Design review of the part built by this model. Coordinates are the model's own, in mm. A direction names the side the tool comes from. Give positions to 0.01 mm unless a question says otherwise; leave off trailing zeros. Write each loop counter-clockwise with the first axis right and the second up, starting at its lowest first coordinate (ties: lowest second). Pieces come first, ordered by that corner, then holes. Notation, with made-up numbers: (-21, 24) - (37, 24) arc R26 ccw to (37, 40) - close; hole circle Ø1 at (0.25, -12.75). An arc over 180 degrees is marked (long way). Write each question's results on one line, items separated by ' | '. Start each with the question number.
from build123d import *

# Parameters (mm, degrees)
BOSS_EXTRUDE1_DEPTH     = 20
CUT_EXTRUDE1_DEPTH      = 57
CUT_EXTRUDE2_START      = -57
CUT_EXTRUDE2_DEPTH      = 57
SKETCH12_W              = 70.48528137
SKETCH12_H              = 6
CUT_EXTRUDE3_DEPTH      = 20
CUT_EXTRUDE4_DEPTH      = 104.740847077
CUT_EXTRUDE4_DEPTH_BACK = 15
SKETCH12_7_OUTSIDE_W    = 149.586
SKETCH12_7_OUTSIDE_H    = 49.586
SKETCH12_7_OUTSIDE_W_2  = 70.48528137
SKETCH12_7_OUTSIDE_H_2  = 3
SKETCH16_W              = 25.2
SKETCH16_H              = 5
CUT_EXTRUDE8_DEPTH      = 57
SKETCH18_R              = 1.4
CUT_EXTRUDE11_DEPTH     = 10
FILLET2_R               = 1
FILLET3_R               = 1.5
SKETCH20_W              = 25.2
SKETCH20_H              = 5
CUT_EXTRUDE12_DEPTH     = 57
FILLET5_R               = 3
FILLET6_R               = 4
SKETCH21_R              = 1.4
CUT_EXTRUDE13_DEPTH     = 20


with BuildPart() as part:
    # Sketch2 → Boss-Extrude1 (new body)
    with BuildSketch(Plane(origin=(0, 0, 0), x_dir=(1, 0, 0), z_dir=(0, 1, 0))):
        Polygon((-41.659950522, -21.859673837), (-41.659950522, -66.859673837), (78.340049478, -66.859673837), (78.340049478, -21.859673837), (53.582690163, -21.859673837), (53.582690163, -1.859673837), (-16.902591207, -1.859673837), (-16.902591207, -21.859673837), align=None)
    extrude(amount=BOSS_EXTRUDE1_DEPTH)

    # Sketch3 → Cut-Extrude1 (cut)
    with BuildSketch(Plane(origin=(78.340049478, 0, 0), x_dir=(0, 0, -1), z_dir=(1, 0, 0))):
        with BuildLine():
            ThreePointArc((-55.925139673, 20), (-46.912626096, 2.661343883), (-31.759673837, 15))
            ThreePointArc((-31.759673837, 15), (-32.02101772, 17.552952259), (-32.794208001, 20))
            Line((-32.794208001, 20), (-55.925139673, 20))
        make_face()
        with BuildLine():
            Line((-55.925139673, 20), (-32.794208001, 20))
            ThreePointArc((-32.794208001, 20), (-44.359673837, 27.6), (-55.925139673, 20))
        make_face()
    extrude(amount=-CUT_EXTRUDE1_DEPTH, mode=Mode.SUBTRACT)

    # Sketch5 → Cut-Extrude2 (cut)
    with BuildSketch(Plane.ZY.offset(41.659950522).offset(CUT_EXTRUDE2_START)):
        with BuildLine():
            ThreePointArc((32.794208001, 20), (41.806721579, 2.661343883), (56.959673837, 15))
            ThreePointArc((56.959673837, 15), (56.698329954, 17.552952259), (55.925139673, 20))
            Line((55.925139673, 20), (32.794208001, 20))
        make_face()
        with BuildLine():
            Line((32.794208001, 20), (55.925139673, 20))
            ThreePointArc((55.925139673, 20), (44.359673837, 27.6), (32.794208001, 20))
        make_face()
    extrude(amount=CUT_EXTRUDE2_DEPTH, mode=Mode.SUBTRACT)

    # Sketch12 → Cut-Extrude3 (cut)
    with BuildSketch(Plane(origin=(0, 0, 1.859673837), x_dir=(-1, 0, 0), z_dir=(0, 0, -1))):
        with Locations((-18.340049478, 17)):
            Rectangle(SKETCH12_W, SKETCH12_H)
    extrude(amount=-CUT_EXTRUDE3_DEPTH, mode=Mode.SUBTRACT)

    # Sketch12_7 outside → Cut-Extrude4 (cut, two sides: drawn at the far end of the back side and taken through both)
    with BuildSketch(Plane(origin=(0, 0, 1.859673837), x_dir=(-1, 0, 0), z_dir=(0, 0, -1)).offset(-CUT_EXTRUDE4_DEPTH_BACK)):
        with Locations((-18.34, 10)):
            Rectangle(SKETCH12_7_OUTSIDE_W, SKETCH12_7_OUTSIDE_H)
        with Locations((-18.340049478, 1.5)):
            Rectangle(SKETCH12_7_OUTSIDE_W_2, SKETCH12_7_OUTSIDE_H_2, mode=Mode.SUBTRACT)
        with Locations((-18.340049478, 12.5)):
            Rectangle(SKETCH12_7_OUTSIDE_W_2, SKETCH12_7_OUTSIDE_H_2, mode=Mode.SUBTRACT)
    extrude(amount=CUT_EXTRUDE4_DEPTH + CUT_EXTRUDE4_DEPTH_BACK, mode=Mode.SUBTRACT)

    # Sketch16 → Cut-Extrude8 (cut)
    with BuildSketch(Plane.ZY.offset(41.659950522)):
        with Locations((44.359673837, 17.5)):
            Rectangle(SKETCH16_W, SKETCH16_H)
    extrude(amount=-CUT_EXTRUDE8_DEPTH, mode=Mode.SUBTRACT)

    # Sketch18 → Cut-Extrude11 (cut)
    with BuildSketch(Plane(origin=(0, 20, 0), x_dir=(1, 0, 0), z_dir=(0, 1, 0))):
        with Locations(Location((-31.659950522, -26.259673837, 0), (0, 0, 270))):
            Circle(SKETCH18_R)
        with Locations(Location((-1.659950522, -26.259673837, 0), (0, 0, 90))):
            Circle(SKETCH18_R)
        with Locations(Location((-1.659950522, -62.459673837, 0), (0, 0, 270))):
            Circle(SKETCH18_R)
        with Locations(Location((-31.659950522, -62.459673837, 0), (0, 0, 90))):
            Circle(SKETCH18_R)
        with Locations(Location((38.340049478, -62.459673837, 0), (0, 0, 90))):
            Circle(SKETCH18_R)
        with Locations(Location((68.340049478, -62.459673837, 0), (0, 0, 270))):
            Circle(SKETCH18_R)
        with Locations(Location((38.340049478, -26.259673837, 0), (0, 0, 270))):
            Circle(SKETCH18_R)
        with Locations(Location((68.340049478, -26.259673837, 0), (0, 0, 90))):
            Circle(SKETCH18_R)
    extrude(amount=-CUT_EXTRUDE11_DEPTH, mode=Mode.SUBTRACT)

    # Fillet2
    fillet2_edges = [part.edges().sort_by_distance(p)[0] for p in [
        (18.340049478, 11, 16.859673837),
        (18.340049478, 3, 16.859673837),
    ]]
    fillet(fillet2_edges, radius=FILLET2_R)

    # Fillet3
    fillet3_edges = [part.edges().sort_by_distance(p)[0] for p in [
        (18.340049478, 11, 1.859673837),
        (18.340049478, 3, 1.859673837),
    ]]
    fillet(fillet3_edges, radius=FILLET3_R)

    # Sketch20 → Cut-Extrude12 (cut)
    with BuildSketch(Plane(origin=(78.340049478, 0, 0), x_dir=(0, 0, -1), z_dir=(1, 0, 0))):
        with Locations((-44.359673837, 17.5)):
            Rectangle(SKETCH20_W, SKETCH20_H)
    extrude(amount=-CUT_EXTRUDE12_DEPTH, mode=Mode.SUBTRACT)

    # Fillet5
    fillet5_edges = [part.edges().sort_by_distance(p)[0] for p in [
        (-41.659950522, 10, 21.859673837),
        (-41.659950522, 10, 66.859673837),
        (78.340049478, 10, 66.859673837),
        (78.340049478, 10, 21.859673837),
    ]]
    fillet(fillet5_edges, radius=FILLET5_R)

    # Fillet6
    fillet6_edges = [part.edges().sort_by_distance(p)[0] for p in [
        (-16.902591207, 7, 21.859673837),
        (53.582690163, 7, 21.859673837),
        (18.340049478, 14, 21.859673837),
    ]]
    fillet(fillet6_edges, radius=FILLET6_R)

    # Sketch21 → Cut-Extrude13 (cut)
    with BuildSketch(Plane(origin=(0, 14, 0), x_dir=(1, 0, 0), z_dir=(0, 1, 0))):
        with Locations(Location((38.340049478, -9.359673837, 0), (0, 0, 270))):
            Circle(SKETCH21_R)
        with Locations(Location((-1.659950522, -9.359673837, 0), (0, 0, 270))):
            Circle(SKETCH21_R)
    extrude(amount=-CUT_EXTRUDE13_DEPTH, mode=Mode.SUBTRACT)


solid = part.part
Q1. Add section C-C on z = 50. State the section outline as (x, y) points, plus the area to 3 significant figures.
Q2. For line 1 along Z through (x, y) = (68.5, 15); line 2 along Z through (x, y) = (38, 16.75); line 3 along Z through (x, y) = (30.5, 8), list the stretches that pass through material, from the lowest coordinate up. Write a range as [from, to].
Q3. Add section A-A on z = 6. State the section outline as (x, y) points, plus the area to 3 significant figures.
Q4. Insertion check: P1, Ø1.7, axis at x = 38.34, z = 9.36, coming from the -Y side (3 decimals); P2, Ø6, axis at y = 11.5, z = 39, coming from the +X side; P3, Ø10, axis at x = 38, y = 7, coming from the -Z side; P4, Ø2, axis at y = 15.5, z = 35.5, coming from the -X side. Each pin has a flat end and moves straight along its axis. Give the tip position at first contact, or say it passes through.
Q5. Add section B-B on x = 22.5. State the section outline as (y, z) points, plus the area to 3 significant figures.
Q6. The part is to be moulded in two halves that separate along Z. For faces 1 (the face through (50, 17, 31.76)), 2 (the face through (-18.105, 7.126, 20.719)), 3 (the face through (77.48, 10.14, 65.96)), say which applies: +Z half, -Z half, draft (parallel to the pull), parting line (faces both ways), or undercut.
Q7. Machinability: for faces 4 (the face through (53.583, 12, 10)), 5 (the face through (39.7, 15.1, 62.8)), 6 (the face through (-12.761, 2.403, 44.083)), 7 (the face through (19, 11, 10)), which of the approach directions +Z, -Z, +X, -X, +Y, -Y give a long, thin tool a straight path to every point of the face, cutting with its end or side? Answer none if there is none.
Result:
1) outline: (-41.66, 0) - (78.34, 0) - (78.34, 3.73) - (21.34, 3.73) - (21.34, 20) - (15.34, 20) - (15.34, 3.73) - (-41.66, 3.73) - close | area: 546 mm²
2) line 1: z = [21.86, 24.87], [27.65, 31.76], [56.96, 61.07], [63.85, 66.86] | line 2: z = [21.66, 24.9], [27.62, 31.76], [56.96, 61.1], [63.82, 66.86] | line 3: z = [16.86, 33.88], [54.84, 66.86]
3) outline: (-16.9, 0) - (53.58, 0) - (53.58, 3) - (-16.9, 3) - close; (-16.9, 11) - (53.58, 11) - (53.58, 14) - (-16.9, 14) - close | area: 423 mm²
4) P1: passes through | P2: stops at x = 21.34 | P3: stops at z = 1.95 | P4: stops at x = 15.34
5) outline: (0, 1.86) - (1.5, 1.86) arc R1.5 ccw to (3, 3.36) - (3, 15.86) arc R1 cw to (4, 16.86) - (10, 16.86) arc R1 cw to (11, 15.86) - (11, 3.36) arc R1.5 ccw to (12.5, 1.86) - (14, 1.86) - (14, 17.86) arc R4 cw to (18, 21.86) - (20, 21.86) - (20, 31.76) - (15, 31.76) arc R12.6 cw to (15, 56.96) - (20, 56.96) - (20, 66.86) - (0, 66.86) - close | area: 688 mm²
6) face 1: undercut | face 2: -Z half | face 3: +Z half
7) face 4: -Z, +X, +Y, -Y | face 5: +Y | face 6: -X, +Y | face 7: -Z, +X, -X
